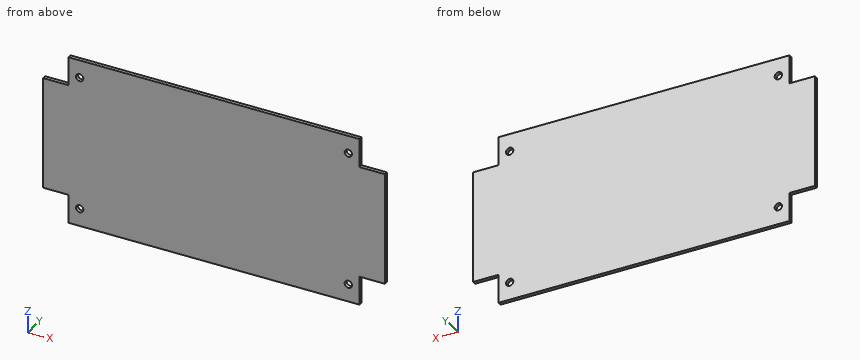
from build123d import *

# Parameters (mm, degrees)
EXTRUDE_1_DEPTH     = 1.5
SKETCH_2_R          = 1.5
CUT_EXTRUDE_2_DEPTH = 1.5


with BuildPart() as part:
    # Эскиз1 → Бобышка-Вытянуть1 (new body)
    with BuildSketch(Plane(origin=(0, 0, 0), x_dir=(1, 0, 0), z_dir=(0, 1, 0))):
        Polygon((-59.5, 34.75), (59.5, 34.75), (59.5, 23), (70, 23), (70, -23), (59.5, -23), (59.5, -34.75), (-59.5, -34.75), (-59.5, -23), (-70, -23), (-70, 23), (-59.5, 23), align=None)
    extrude(amount=EXTRUDE_1_DEPTH)

    # Эскиз2 → Вырез-Вытянуть2 (cut)
    with BuildSketch(Plane(origin=(0, 0, 0), x_dir=(1, 0, 0), z_dir=(0, 1, 0))):
        with Locations(Location((-55, 27.5, 0), (0, 0, 270))):
            Circle(SKETCH_2_R)
        with Locations(Location((-55, -27.5, 0), (0, 0, 270))):
            Circle(SKETCH_2_R)
        with Locations(Location((55, -27.5, 0), (0, 0, 270))):
            Circle(SKETCH_2_R)
        with Locations(Location((55, 27.5, 0), (0, 0, 270))):
            Circle(SKETCH_2_R)
    extrude(amount=CUT_EXTRUDE_2_DEPTH, mode=Mode.SUBTRACT)


solid = part.part
Could you check a few things on this model? Use its own coordinates, in mm. Give positions to 0.01 mm unless a question says otherwise; leave off trailing zeros. Order: outer loops, then holes, each group sorted by start corner. A loop starts at its lowest first (then second) coordinate and runs counter-clockwise, first axis right, second up.
1. Will these pins go through, and if not, where does the flat tip stop? P1, Ø0.8, axis at y = 1, z = -31, coming from the +X side; P2, Ø0.8, axis at x = -63.5, y = 0.5, coming from the -Z side; P3, Ø0.8, axis at x = 67, y = 1, coming from the +Z side; P4, Ø2.5, axis at x = -55, z = -27.5, coming from the +Y side.
2. Suppose I cut it at B-B (x = 55). List the corners of the cut face in (y, z) for me.
3. Suppose I cut it at A-A (z = 27.5). List the corners of the cut face in (x, y) for me.
4. I need wall thicknesses on L1, parallel to X at y = 0.45, z = 27.5; L2, parallel to X at y = 1.3, z = 27; L3, parallel to X at y = 0.65, z = 30.5. Which ranges of each line are inside material? Lowest first, please.
5. Suppose I cut it at C-C (y = 0.8). List the corners of the cut face in (x, z) for me.
Solved:
1. P1: stops at x = 59.5
1. P2: stops at z = -23
1. P3: stops at z = 23
1. P4: passes through
2. outline: (0, -34.75) - (1.5, -34.75) - (1.5, -29) - (0, -29) - close; (0, -26) - (1.5, -26) - (1.5, 26) - (0, 26) - close; (0, 29) - (1.5, 29) - (1.5, 34.75) - (0, 34.75) - close
3. outline: (-59.5, 0) - (-56.5, 0) - (-56.5, 1.5) - (-59.5, 1.5) - close; (-53.5, 0) - (53.5, 0) - (53.5, 1.5) - (-53.5, 1.5) - close; (56.5, 0) - (59.5, 0) - (59.5, 1.5) - (56.5, 1.5) - close
4. L1: x = -59.5 to -56.5, -53.5 to 53.5, 56.5 to 59.5
4. L2: x = -59.5 to -56.41, -53.59 to 53.59, 56.41 to 59.5
4. L3: x = -59.5 to 59.5
5. outline: (-70, -23) - (-59.5, -23) - (-59.5, -34.75) - (59.5, -34.75) - (59.5, -23) - (70, -23) - (70, 23) - (59.5, 23) - (59.5, 34.75) - (-59.5, 34.75) - (-59.5, 23) - (-70, 23) - close; hole circle Ø3 at (-55, -27.5); hole circle Ø3 at (-55, 27.5); hole circle Ø3 at (55, -27.5); hole circle Ø3 at (55, 27.5)
